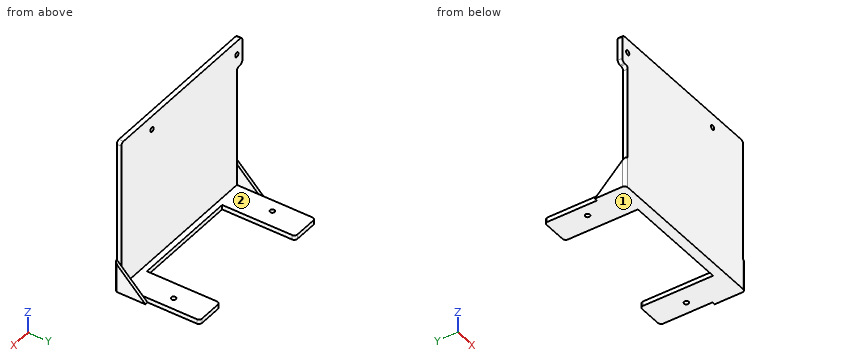
from build123d import *

# Parameters (mm, degrees)
SKETCH_1_W          = 107.5
SKETCH_1_H          = 54
EXTRUDE_1_DEPTH     = 3
SKETCH_2_W          = 107.5
SKETCH_2_H          = 3
EXTRUDE_2_DEPTH     = 97
SKETCH_4_W          = 5
SKETCH_4_H          = 18
EXTRUDE_3_DEPTH     = 3
SKETCH_5_R          = 1.5
CUT_EXTRUDE_1_DEPTH = 3
SKETCH_6_W          = 70
SKETCH_6_H          = 47.5
CUT_EXTRUDE_2_DEPTH = 3
SKETCH_7_R          = 1.5
CUT_EXTRUDE_3_DEPTH = 3
EXTRUDE_4_DEPTH     = 2
EXTRUDE_5_DEPTH     = 2
FILLET_1_R          = 2
FILLET_2_R          = 2


with BuildPart() as part:
    # 草图1 → 凸台-拉伸1 (new body)
    with BuildSketch(Plane.XY):
        with Locations((0, 27)):
            Rectangle(SKETCH_1_W, SKETCH_1_H)
    extrude(amount=EXTRUDE_1_DEPTH)

    # 草图2 → 凸台-拉伸2 (add)
    with BuildSketch(Plane.XY.offset(3)):
        with Locations((0, 1.5)):
            Rectangle(SKETCH_2_W, SKETCH_2_H)
    extrude(amount=EXTRUDE_2_DEPTH)

    # 草图4 → 凸台-拉伸3 (add)
    with BuildSketch(Plane(origin=(0, 3, 0), x_dir=(1, 0, 0), z_dir=(0, 1, 0))):
        with Locations((-56.25, -91)):
            Rectangle(SKETCH_4_W, SKETCH_4_H)
    extrude(amount=-EXTRUDE_3_DEPTH)

    # 草图5 → 切除-拉伸1 (cut)
    with BuildSketch(Plane(origin=(0, 3, 0), x_dir=(1, 0, 0), z_dir=(0, 1, 0))):
        with Locations(Location((-53.75, -91, 0), (0, 0, 180))):
            Circle(SKETCH_5_R)
        with Locations(Location((25.25, -91, 0), (0, 0, 180))):
            Circle(SKETCH_5_R)
    extrude(amount=-CUT_EXTRUDE_1_DEPTH, mode=Mode.SUBTRACT)

    # 草图6 → 切除-拉伸2 (cut)
    with BuildSketch(Plane.XY.offset(3)):
        with Locations((0, 30.25)):
            Rectangle(SKETCH_6_W, SKETCH_6_H)
    extrude(amount=-CUT_EXTRUDE_2_DEPTH, mode=Mode.SUBTRACT)

    # 草图7 → 切除-拉伸3 (cut)
    with BuildSketch(Plane.XY.offset(3)):
        with Locations((46, 31.5)):
            Circle(SKETCH_7_R)
        with Locations((-46, 31.5)):
            Circle(SKETCH_7_R)
    extrude(amount=-CUT_EXTRUDE_3_DEPTH, mode=Mode.SUBTRACT)

    # 草图8 → 凸台-拉伸4 (add)
    with BuildSketch(Plane.ZY.offset(53.75)):
        Polygon((0, 0), (20, 0), (0, 20), align=None)
    extrude(amount=EXTRUDE_4_DEPTH)

    # 草图9 → 凸台-拉伸5 (add)
    with BuildSketch(Plane(origin=(53.75, 0, 0), x_dir=(0, 0, -1), z_dir=(1, 0, 0))):
        Polygon((0, 0), (0, 20), (-20, 0), align=None)
    extrude(amount=EXTRUDE_5_DEPTH)

    # 圆角1
    fillet_1_edges = [part.edges().sort_by_distance(p)[0] for p in [
        (-55.75, 0, 10),
        (55.75, 0, 10),
        (53.75, 54, 1.5),
        (35, 54, 1.5),
        (-35, 54, 1.5),
        (-53.75, 54, 1.5),
    ]]
    fillet(fillet_1_edges, radius=FILLET_1_R)

    # 圆角2
    fillet_2_edges = [part.edges().sort_by_distance(p)[0] for p in [
        (53.75, 1.5, 100),
        (-53.75, 1.5, 82),
        (-58.75, 1.5, 100),
        (-58.75, 1.5, 82),
    ]]
    fillet(fillet_2_edges, radius=FILLET_2_R)


solid = part.part
Design review of the part built by this model. Coordinates are the model's own, in mm. Face numbers are marked on the shaded views. Coordinates: 2 decimals unless noted, no trailing zeros. Loops run counter-clockwise (first coordinate to the right, second up) from the corner with the lowest first, then second, coordinate; pieces in that order, holes last.
Item 1: Add section D-D (y = 11.5). Write out the cut boundary in (x, z), and give its area (4 significant figures).
Completed:
outline: (-55.75, 0) - (-35, 0) - (-35, 3) - (-53.75, 3) - (-53.75, 8.5) - (-55.75, 8.5) - close; (35, 0) - (55.75, 0) - (55.75, 8.5) - (53.75, 8.5) - (53.75, 3) - (35, 3) - close
area: 146.5 mm2
Item 2: Add section B-B (y = 31.5). Write out the cut boundary in (x, z).
Completed:
outline: (-53.75, 0) - (-47.5, 0) - (-47.5, 3) - (-53.75, 3) - close; (-44.5, 0) - (-35, 0) - (-35, 3) - (-44.5, 3) - close; (35, 0) - (44.5, 0) - (44.5, 3) - (35, 3) - close; (47.5, 0) - (53.75, 0) - (53.75, 3) - (47.5, 3) - close
Item 3: Draft analysis for pull direction X (two halves, no side actions). For the marked faces 1 and 2, state which applies: pulls with the +X half, pulls with the -X half, needs draft (parallel to the pull), parting line crosses it, or undercut.
Completed:
face 1: needs draft
face 2: undercut
Item 4: Wall thickness on L1, parallel to X at y = 1.5, z = 91; L2, parallel to X at y = 31, z = 1; L3, parallel to Y at x = -43, z = 5.5: over which ranges is each line inside the solid? List them lowest first.
Completed:
L1: x = -58.75 to -55.25, -52.25 to 23.75, 26.75 to 53.75
L2: x = -53.75 to -47.41, -44.59 to -35, 35 to 44.59, 47.41 to 53.75
L3: y = 0 to 3
Item 5: Add section A-A (x = 25.25). Write out the cut boundary in (y, z).
Completed:
outline: (0, 0) - (6.5, 0) - (6.5, 3) - (3, 3) - (3, 89.5) - (0, 89.5) - close; (0, 92.5) - (3, 92.5) - (3, 100) - (0, 100) - close
Item 6: Add section C-C (z = 91). Write out the cut boundary in (x, y), and give its area (4 significant figures).
Completed:
outline: (-58.75, 0) - (-55.25, 0) - (-55.25, 3) - (-58.75, 3) - close; (-52.25, 0) - (23.75, 0) - (23.75, 3) - (-52.25, 3) - close; (26.75, 0) - (53.75, 0) - (53.75, 3) - (26.75, 3) - close
area: 319.5 mm2
Item 7: Clearance check with flat-ended pins moving along their axes: pin 1 (5 mm diameter, centred on x = -23.5, y = 9.5, fed in from +Z); pin 2 (2 mm diameter, centred on x = -19, z = 41.5, fed in from +Y); pin 3 (0.9 mm diameter, centred on y = 33.5, z = 1.5, fed in from -X); pin 4 (4 mm diameter, centred on x = -46, y = 31.5, fed in from +Z). State where each tip first meets the part, or that it passes through.
Completed:
pin 1: passes through
pin 2: stops at y = 3
pin 3: stops at x = -53.75
pin 4: stops at z = 3
